Input: part model. Units: mm. Frame: model coordinates. Face numbers are marked on the shaded views. A direction names the side the tool comes from. Round coordinates to 2 decimals unless told otherwise and drop trailing zeros. Loops run counter-clockwise (first coordinate to the right, second up) from the corner with the lowest first, then second, coordinate; pieces in that order, holes last.
(1) Line query: line 1 (Y direction, x = -40, z = -2.75); line 2 (Z direction, x = -17, y = 42); line 3 (X direction, y = 31, z = -6). Output: solid intervals per line, ascending.
(2) Access query for the marked faces 1 and 2. Directions: +Z, -Z, +X, -X, +Y, -Y. A direction counts if a zero-diameter tool reaches every point of the face in a straight line with its end or side. Return the directions, or none.
(3) First-contact query: pin 1 Ø15.5 at (x, y) = (-33, 53) entering from -Z; pin 2 Ø1 at (y, z) = (40.5, -37.5) entering from -X; pin 3 Ø1 at (y, z) = (13.5, -14) entering from -X; pin 4 Ø1.5 at (y, z) = (11, -40.5) entering from -X. Flat tips, straight axial feed; report the tip coordinate or a pass-through.
(4) Cut plane A-A, the plane y = 20. Output: boundary loops of the cut face in (x, z).
(5) Draft query along Y for the marked faces 3, 4 and 5. Return one class per face: released by +Y, released by -Y, zero draft, split by the parting line, or undercut.
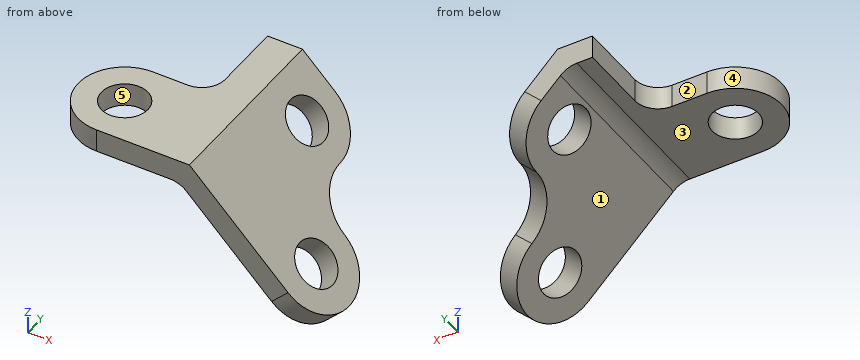
from build123d import *

# Parameters (mm, degrees)
SKETCH_1_R      = 10
EXTRUDE_1_DEPTH = 10
SKETCH_2_R      = 10
EXTRUDE_2_DEPTH = 10
FILLET_1_R      = 10


with BuildPart() as part:
    # 草圖1 → 填料-伸長1 (new body)
    with BuildSketch(Plane.XY):
        with BuildLine():
            Line((0, 80), (0, 0))
            Line((0, 0), (-40, 0))
            ThreePointArc((-40, 0), (-60, 20), (-40, 40))
            Line((-40, 40), (-25, 40))
            ThreePointArc((-25, 40), (-17.928932188, 42.928932188), (-15, 50))
            Line((-15, 50), (-15, 80))
            Line((-15, 80), (0, 80))
        make_face()
        with Locations((-40, 20)):
            Circle(SKETCH_1_R, mode=Mode.SUBTRACT)
    extrude(amount=-EXTRUDE_1_DEPTH)

    # 草圖2 → 填料-伸長2 (add)
    with BuildSketch(Plane(origin=(0, 0, 0), x_dir=(0, -1, 0), z_dir=(0.707106781, 0, 0.707106781))):
        with BuildLine():
            Line((0, 60), (0, 0))
            Line((0, 0), (-80, 0))
            Line((-80, 0), (-80, 20))
            ThreePointArc((-80, 20), (-74.142135624, 34.142135624), (-60, 40))
            ThreePointArc((-60, 40), (-45.857864376, 45.857864376), (-40, 60))
            ThreePointArc((-40, 60), (-20, 80), (0, 60))
        make_face()
        with Locations((-60, 20)):
            Circle(SKETCH_2_R, mode=Mode.SUBTRACT)
        with Locations((-20, 60)):
            Circle(SKETCH_2_R, mode=Mode.SUBTRACT)
    extrude(amount=-EXTRUDE_2_DEPTH)

    # 圓角1
    fillet_1_edges = [part.edges().sort_by_distance(p)[0] for p in [
        (-4.142135624, 40, -10),
    ]]
    fillet(fillet_1_edges, radius=FILLET_1_R)


solid = part.part
Reported:
1. line 1: y = 0 to 10, 30 to 40
1. line 2: z = -10 to 0
1. line 3: x = -56.7 to 6
2. face 1: -Z, -X, +Y, -Y
2. face 2: +Z, -Z, -X, +Y
3. pin 1: passes through
3. pin 2: stops at x = 22.86
3. pin 3: stops at x = -0.64
3. pin 4: stops at x = 25.61
4. outline: (-60, -10) - (-50, -10) - (-50, 0) - (-60, 0) - close; (-30, -10) - (-8.28, -10) arc R10 cw to (-1.21, -12.93) - (28.28, -42.43) - (35.36, -35.36) - (0, 0) - (-30, 0) - close; (42.43, -56.57) - (49.5, -63.64) - (56.57, -56.57) - (49.5, -49.5) - close
5. face 3: zero draft
5. face 4: split by the parting line
5. face 5: undercut
